Part model, mm, in its own coordinate system. A direction names the side the tool comes from. Give positions to 0.01 mm unless a question says otherwise; leave off trailing zeros. Write each loop counter-clockwise with the first axis right and the second up, starting at its lowest first coordinate (ties: lowest second). Pieces come first, ordered by that corner, then holes.
from build123d import *

# Parameters (mm, degrees)
SKETCH_1_R          = 2.15
EXTRUDE_1_DEPTH     = 2
SKETCH_2_W          = 23.301883536
SKETCH_2_H          = 5.8
SKETCH_2_W_2        = 10.898116464
EXTRUDE_2_DEPTH     = 1.6
FILLET_1_R          = 1
CHAMFER_START       = -66
CHAMFER_1_OUTLINE_W = 25
CHAMFER_1_OUTLINE_H = 4
CHAMFER_1_DEPTH     = 4.467828672
FILLET_2_R          = 1
FILLET_3_R          = 20
FILLET_5_R          = 0.4
FILLET_6_R          = 0.4


with BuildPart() as part:
    # 草图1 → 凸台-拉伸1 (new body)
    with BuildSketch(Plane.XY):
        with BuildLine():
            Line((-61.382701422, 26.657582938), (-53.382701422, 26.657582938))
            Line((-53.382701422, 26.657582938), (-53.382701422, -34.342417062))
            Line((-53.382701422, -34.342417062), (-61.382701422, -34.342417062))
            Line((-61.382701422, -34.342417062), (-93.382701422, -34.342417062))
            Line((-93.382701422, -34.342417062), (-93.382701422, -14.342417062))
            Line((-93.382701422, -14.342417062), (-81.382701422, -14.342417062))
            ThreePointArc((-81.382701422, -14.342417062), (-67.240565798, -8.484552685), (-61.382701422, 5.657582938))
            Line((-61.382701422, 5.657582938), (-61.382701422, 26.657582938))
        make_face()
        with Locations((-79.650533319, -24.342417062)):
            Circle(SKETCH_1_R, mode=Mode.SUBTRACT)
    extrude(amount=EXTRUDE_1_DEPTH)

    # 草图2 → 凸台-拉伸2 (add)
    with BuildSketch(Plane(origin=(0, 0, 0), x_dir=(-1, 0, 0), z_dir=(0, 0, -1))):
        with Locations((65.099591551, -24.342417062)):
            Rectangle(SKETCH_2_W, SKETCH_2_H)
        with Locations((87.999591551, -24.342417062)):
            Rectangle(SKETCH_2_W_2, SKETCH_2_H)
    extrude(amount=EXTRUDE_2_DEPTH)

    # 圆角1
    fillet_1_edges = [part.edges().sort_by_distance(p)[0] for p in [
        (-53.382701422, 26.657582938, 1),
        (-53.382701422, -34.342417062, 1),
        (-93.382701422, -34.342417062, 1),
        (-93.382701422, -14.342417062, 1),
    ]]
    fillet(fillet_1_edges, radius=FILLET_1_R)

    # 倒角1: read off the stored shape, not the designer's step
    # 倒角1 outline → 倒角1 (cut)
    with BuildSketch(Plane(origin=(0, 0, 0), x_dir=(0.13944684527210205, 0.9902295579024383, 0), z_dir=(0.9902295579024384, -0.13944684527210205, 0)).offset(CHAMFER_START)):
        with Locations((7.5, 1)):
            Rectangle(CHAMFER_1_OUTLINE_W, CHAMFER_1_OUTLINE_H)
    extrude(amount=CHAMFER_1_DEPTH, mode=Mode.SUBTRACT)

    # 圆角2
    fillet_2_edges = [part.edges().sort_by_distance(p)[0] for p in [
        (-58.385305734, 26.657582938, 1),
    ]]
    fillet(fillet_2_edges, radius=FILLET_2_R)

    # 圆角3
    fillet_3_edges = [part.edges().sort_by_distance(p)[0] for p in [
        (-61.384966041, 5.356618447, 1),
    ]]
    fillet(fillet_3_edges, radius=FILLET_3_R)

    # 圆角5
    # the kernel refuses this fillet: 0.4 mm, written as the material it takes off along each edge
    with BuildSketch(Plane(origin=(-93.382701422, -21.442417062, 0), x_dir=(1, 0, 0), z_dir=(0, 1, 0)), Plane(origin=(-93.382701422, -33.342417062, 0), x_dir=(1, 0, 0), z_dir=(0, 1, 0))) as fillet_5_piece_1:
        with BuildLine():
            CenterArc((FILLET_5_R, -FILLET_5_R), FILLET_5_R, 90, 90)
            Line((0, -FILLET_5_R), (0, 0))
            Line((0, 0), (FILLET_5_R, 0))
        make_face()
    extrude(amount=6.1, mode=Mode.SUBTRACT)
    with BuildSketch(Plane(origin=(-92.382701422, -15.342417062, 0), x_dir=(0, 1, 0), z_dir=(1, 0, 0))) as fillet_5_piece_2:
        with BuildLine():
            CenterArc((1 - FILLET_5_R, FILLET_5_R), FILLET_5_R, 270, 90)
            Line((1, FILLET_5_R), (1, 0))
            Line((1, 0), (1 - FILLET_5_R, 0))
        make_face()
    revolve(axis=Axis((-92.382701422, -15.342417062, 0), (0, 0, 1)), revolution_arc=90, mode=Mode.SUBTRACT)
    with BuildSketch(Plane(origin=(-92.382701422, -14.342417062, 0), x_dir=(0, -1, 0), z_dir=(1, 0, 0))) as fillet_5_piece_3:
        with BuildLine():
            CenterArc((FILLET_5_R, -FILLET_5_R), FILLET_5_R, 90, 90)
            Line((0, -FILLET_5_R), (0, 0))
            Line((0, 0), (FILLET_5_R, 0))
        make_face()
    extrude(amount=11, mode=Mode.SUBTRACT)
    with BuildSketch(Plane(origin=(-81.382701422, 5.657582938, 0), x_dir=(0, -1, 0), z_dir=(-1, 0, 0))) as fillet_5_piece_4:
        with BuildLine():
            CenterArc((20 + FILLET_5_R, FILLET_5_R), FILLET_5_R, 180, 90)
            Line((20, FILLET_5_R), (20, 0))
            Line((20, 0), (20 + FILLET_5_R, 0))
        make_face()
    revolve(axis=Axis((-81.382701422, 5.657582938, 0), (0, 0, 1)), revolution_arc=87.040880974, mode=Mode.SUBTRACT)
    with BuildSketch(Plane(origin=(-92.382701422, -33.342417062, 0), x_dir=(-1, 0, 0), z_dir=(0, 1, 0))) as fillet_5_piece_5:
        with BuildLine():
            CenterArc((1 - FILLET_5_R, FILLET_5_R), FILLET_5_R, 270, 90)
            Line((1, FILLET_5_R), (1, 0))
            Line((1, 0), (1 - FILLET_5_R, 0))
        make_face()
    revolve(axis=Axis((-92.382701422, -33.342417062, 0), (0, 0, 1)), revolution_arc=90, mode=Mode.SUBTRACT)
    with BuildSketch(Plane(origin=(-92.382701422, -34.342417062, 0), x_dir=(0, 1, 0), z_dir=(1, 0, 0))) as fillet_5_piece_6:
        with BuildLine():
            CenterArc((FILLET_5_R, FILLET_5_R), FILLET_5_R, 180, 90)
            Line((0, FILLET_5_R), (0, 0))
            Line((0, 0), (FILLET_5_R, 0))
        make_face()
    extrude(amount=38, mode=Mode.SUBTRACT)
    with BuildSketch(Plane(origin=(-54.382701422, -33.342417062, 0), x_dir=(0, -1, 0), z_dir=(-1, 0, 0))) as fillet_5_piece_7:
        with BuildLine():
            CenterArc((1 - FILLET_5_R, FILLET_5_R), FILLET_5_R, 270, 90)
            Line((1, FILLET_5_R), (1, 0))
            Line((1, 0), (1 - FILLET_5_R, 0))
        make_face()
    revolve(axis=Axis((-54.382701422, -33.342417062, 0), (0, 0, 1)), revolution_arc=90, mode=Mode.SUBTRACT)
    with BuildSketch(Plane(origin=(-53.382701422, 25.657582938, 0), x_dir=(-1, 0, 0), z_dir=(0, -1, 0))) as fillet_5_piece_8_section:
        with BuildLine():
            CenterArc((FILLET_5_R, -FILLET_5_R), FILLET_5_R, 90, 90)
            Line((0, -FILLET_5_R), (0, 0))
            Line((0, 0), (FILLET_5_R, 0))
        make_face()
    fillet_5_piece_8 = extrude(amount=59, mode=Mode.PRIVATE)
    fillet_5_piece_8 = split(fillet_5_piece_8, bisect_by=Plane(origin=(-53.382701422, -21.442417062, 0), z_dir=(0, 1, 0)), keep=Keep.TOP, mode=Mode.PRIVATE)
    add(fillet_5_piece_8, mode=Mode.SUBTRACT)
    with BuildSketch(Plane(origin=(-53.382701422, 25.657582938, 0), x_dir=(-1, 0, 0), z_dir=(0, -1, 0))) as fillet_5_piece_9_section:
        with BuildLine():
            CenterArc((FILLET_5_R, -FILLET_5_R), FILLET_5_R, 90, 90)
            Line((0, -FILLET_5_R), (0, 0))
            Line((0, 0), (FILLET_5_R, 0))
        make_face()
    fillet_5_piece_9 = extrude(amount=59, mode=Mode.PRIVATE)
    fillet_5_piece_9 = split(fillet_5_piece_9, bisect_by=Plane(origin=(-53.448649783, 25.657582938, 0), z_dir=(1, 0, 0)), keep=Keep.TOP, mode=Mode.PRIVATE)
    add(fillet_5_piece_9, mode=Mode.SUBTRACT)
    with BuildSketch(Plane(origin=(-53.382701422, 25.657582938, 0), x_dir=(-1, 0, 0), z_dir=(0, -1, 0))) as fillet_5_piece_10_section:
        with BuildLine():
            CenterArc((FILLET_5_R, -FILLET_5_R), FILLET_5_R, 90, 90)
            Line((0, -FILLET_5_R), (0, 0))
            Line((0, 0), (FILLET_5_R, 0))
        make_face()
    fillet_5_piece_10 = extrude(amount=59, mode=Mode.PRIVATE)
    fillet_5_piece_10 = split(fillet_5_piece_10, bisect_by=Plane(origin=(-53.382701422, -27.242417062, 0), z_dir=(0, -1, 0)), keep=Keep.TOP, mode=Mode.PRIVATE)
    add(fillet_5_piece_10, mode=Mode.SUBTRACT)
    with BuildSketch(Plane(origin=(-54.382701422, 25.657582938, 0), x_dir=(0, 1, 0), z_dir=(-1, 0, 0))) as fillet_5_piece_11:
        with BuildLine():
            CenterArc((1 - FILLET_5_R, -FILLET_5_R), FILLET_5_R, 0, 90)
            Line((1, -FILLET_5_R), (1, 0))
            Line((1, 0), (1 - FILLET_5_R, 0))
        make_face()
    revolve(axis=Axis((-54.382701422, 25.657582938, 0), (0, 0, -1)), revolution_arc=90, mode=Mode.SUBTRACT)
    with BuildSketch(Plane(origin=(-57.516261634, 26.657582938, 0), x_dir=(0, -1, 0), z_dir=(1, 0, 0))) as fillet_5_piece_12:
        with BuildLine():
            CenterArc((FILLET_5_R, -FILLET_5_R), FILLET_5_R, 90, 90)
            Line((0, -FILLET_5_R), (0, 0))
            Line((0, 0), (FILLET_5_R, 0))
        make_face()
    extrude(amount=3.133560212, mode=Mode.SUBTRACT)
    with BuildSketch(Plane(origin=(-57.516261634, 25.657582938, 0), x_dir=(0, 1, 0), z_dir=(1, 0, 0))) as fillet_5_piece_13:
        with BuildLine():
            CenterArc((1 - FILLET_5_R, FILLET_5_R), FILLET_5_R, 270, 90)
            Line((1, FILLET_5_R), (1, 0))
            Line((1, 0), (1 - FILLET_5_R, 0))
        make_face()
    revolve(axis=Axis((-57.516261634, 25.657582938, 0), (0, 0, 1)), revolution_arc=81.984161159, mode=Mode.SUBTRACT)
    with BuildSketch(Plane(origin=(-58.506491192, 25.797029784, 0), x_dir=(0.9902295579024384, -0.13944684527210205, 0), z_dir=(-0.13944684527210205, -0.9902295579024384, 0))) as fillet_5_piece_14:
        with BuildLine():
            CenterArc((FILLET_5_R, FILLET_5_R), FILLET_5_R, 180, 90)
            Line((0, FILLET_5_R), (0, 0))
            Line((0, 0), (FILLET_5_R, 0))
        make_face()
    extrude(amount=19.60701568, mode=Mode.SUBTRACT)
    with BuildSketch(Plane(origin=(-41.436036516, 3.592646409, 0), x_dir=(-0.9902295579024383, 0.13944684527210185, 0), z_dir=(0.13944684527210185, 0.9902295579024383, 0))) as fillet_5_piece_15:
        with BuildLine():
            CenterArc((20 - FILLET_5_R, FILLET_5_R), FILLET_5_R, 270, 90)
            Line((20, FILLET_5_R), (20, 0))
            Line((20, 0), (20 - FILLET_5_R, 0))
        make_face()
    revolve(axis=Axis((-41.436036516, 3.592646409, 0), (0, 0, 1)), revolution_arc=5.056719815, mode=Mode.SUBTRACT)

    # 圆角6
    fillet_6_edges = [part.edges().sort_by_distance(p)[0] for p in [
        (-86.882701422, -14.342417062, 2),
        (-55.949481528, 26.657582938, 2),
        (-53.382701422, -3.842417062, 2),
        (-93.382701422, -24.342417062, 2),
        (-73.382701422, -34.342417062, 2),
        (-93.089808203, -14.63531028, 2),
        (-93.089808203, -34.049523843, 2),
        (-53.675594641, -34.049523843, 2),
        (-53.675594641, 26.36468972, 2),
        (-59.873559433, 16.089306549, 2),
        (-58.172216341, 26.412383192, 2),
        (-67.610435183, -8.844992097, 2),
        (-61.344378918, 5.505210859, 2),
    ]]
    fillet(fillet_6_edges, radius=FILLET_6_R)


solid = part.part
1) Flat gauge pins, fed straight in: P1, Ø1, axis at x = -87, z = -1, coming from the +Y side; P2, Ø0.5, axis at x = -68, z = -0.5, coming from the -Y side; P3, Ø0.5, axis at y = -21, z = 0.5, coming from the -X side. Where does each tip first touch, or does it go through?
Check result:
P1: stops at y = -21.44
P2: stops at y = -27.24
P3: stops at x = -93.38
2) Saw through at A-A (z = -1). Write the cut outline in (x, y), and give its area (3 significant figures).
Check result:
outline: (-93.45, -27.24) - (-82.55, -27.24) - (-82.55, -21.44) - (-93.45, -21.44) - close; (-76.75, -27.24) - (-53.45, -27.24) - (-53.45, -21.44) - (-76.75, -21.44) - close
area: 198 mm2
3) Saw through at D-D (x = -87.5). Write the cut outline in (y, z), and give its area (3 significant figures).
Check result:
outline: (-34.34, 0.4) arc R0.4 ccw to (-33.94, 0) - (-27.24, 0) - (-27.24, -1.6) - (-21.44, -1.6) - (-21.44, 0) - (-14.74, 0) arc R0.4 ccw to (-14.34, 0.4) - (-14.34, 1.6) arc R0.4 ccw to (-14.74, 2) - (-33.94, 2) arc R0.4 ccw to (-34.34, 1.6) - close
area: 49.1 mm2
4) Drill centre lines: L1, parallel to X at y = -23, z = -1; L2, parallel to Y at x = -85.5, z = 0.7; L3, parallel to X at y = -30.5, z = 0.55. Where is each one in solid material? Low to high.
Check result:
L1: x = -93.45 to -82.55, -76.75 to -53.45
L2: y = -34.34 to -14.34
L3: x = -93.38 to -53.38
5) Saw through at C-C (y = -18). Write the cut outline in (x, z).
Check result:
outline: (-93.38, 0.4) arc R0.4 ccw to (-92.98, 0) - (-53.78, 0) arc R0.4 ccw to (-53.38, 0.4) - (-53.38, 1.6) arc R0.4 ccw to (-53.78, 2) - (-92.98, 2) arc R0.4 ccw to (-93.38, 1.6) - close
6) Saw through at B-B (x = -56.5). Write the cut outline in (y, z).
Check result:
outline: (-34.34, 0.4) arc R0.4 ccw to (-33.94, 0) - (-27.24, 0) - (-27.24, -1.6) - (-21.44, -1.6) - (-21.44, 0) - (26.26, 0) arc R0.4 ccw to (26.66, 0.4) - (26.66, 1.6) arc R0.4 ccw to (26.26, 2) - (-33.94, 2) arc R0.4 ccw to (-34.34, 1.6) - close
7) 3-axis set-ups, long thin cutter, end or side, ignore diameter. For faces 1 (the flat face through (-53.449, -24, -1)), 2 (the flat face through (-82.551, -24, -1)), 3 (the flat face through (-87, -14.342, 1)), 4 (the flat face through (-93.383, -24, 1)), 5 (the flat face through (-53.383, -3, 1)): which of +Z, -Z, +X, -X, +Y, -Y reach the whole face in a straight line?
Check result:
face 1: -Z, +X, +Y, -Y
face 2: -Z, +Y, -Y
face 3: +Z, -Z, -X, +Y
face 4: +Z, -X, +Y, -Y
face 5: +Z, -Z, +X, +Y, -Y
